Model file for the job. Use its own axes, mm. Coordinates: 2 decimals unless noted, no trailing zeros. Order: outer loops, then holes, each group sorted by start corner. A loop starts at its lowest first (then second) coordinate and runs counter-clockwise, first axis right, second up. Notation, with made-up numbers: M -10.75,-9.5 L 0.25,-9.5 A36 cw 0.25,28.5 Z; hole C -16,46.25 d2. An arc over 180 degrees is marked long. Return JSON: item names as keys, results as strings.
```python
from build123d import *

# Parameters (mm, degrees)
ESBO_O1_W                                            = 18
ESBO_O1_H                                            = 400
RESSALTO_EXTRUS_O1_DEPTH                             = 3.5
FURO_DE_DI_METRO_2_0_2_1_D                           = 2
FURO_DE_DI_METRO_6_0_6_1_D                           = 6
REBAIXO_PARA_PARAFUSO_DE_M_QUINA_DE_CABE_D           = 3.5
REBAIXO_PARA_PARAFUSO_DE_M_QUINA_DE_CABE_CBORE_D     = 6
REBAIXO_PARA_PARAFUSO_DE_M_QUINA_DE_CABE_CBORE_DEPTH = 3.5
PADR_O_LINEAR1_COUNT                                 = 13
PADR_O_LINEAR1_PITCH                                 = 30
PADR_O_LINEAR2_COUNT                                 = 14
PADR_O_LINEAR2_PITCH                                 = 30
CHANFRO1_SIZE                                        = 0.3


with BuildPart() as part:
    # Esboço1 → Ressalto-extrusão1 (new, symmetric)
    with BuildSketch(Plane.XZ):
        Rectangle(ESBO_O1_W, ESBO_O1_H)
    extrude(amount=RESSALTO_EXTRUS_O1_DEPTH, both=True)

    # Furo de diâmetro Ø2.0 (2)1 (through all)
    with Locations(Plane(origin=(0, 0, -200), x_dir=(-1, 0, 0), z_dir=(0, 0, -1))):
        with Locations((-8.669077014, 4.635653864), (9, 1.2)):
            furo_de_di_metro_2_0_2_1 = Hole(FURO_DE_DI_METRO_2_0_2_1_D / 2)

    # Furo de diâmetro Ø6.0 (6)1 (through all)
    with Locations(Plane(origin=(0, 3.5, 0), x_dir=(1, 0, 0), z_dir=(0, 1, 0))):
        with Locations((0, -175)):
            furo_de_di_metro_6_0_6_1 = Hole(FURO_DE_DI_METRO_6_0_6_1_D / 2)

    # Rebaixo para parafuso de máquina de cabeça sextavada de M31 (through all)
    with Locations(Plane(origin=(0, 3.5, 0), x_dir=(1, 0, 0), z_dir=(0, 1, 0))):
        with Locations((0, -190)):
            rebaixo_para_parafuso_de_m_quina_de_cabe = CounterBoreHole(REBAIXO_PARA_PARAFUSO_DE_M_QUINA_DE_CABE_D / 2, REBAIXO_PARA_PARAFUSO_DE_M_QUINA_DE_CABE_CBORE_D / 2, REBAIXO_PARA_PARAFUSO_DE_M_QUINA_DE_CABE_CBORE_DEPTH)

    # Padrão linear1: Furo de diâmetro Ø6.0 (6)1 ×13
    with Locations(*[(0, 0, -i * PADR_O_LINEAR1_PITCH) for i in range(1, PADR_O_LINEAR1_COUNT)]):
        add(furo_de_di_metro_6_0_6_1, mode=Mode.SUBTRACT)

    # Padrão linear2: Rebaixo para parafuso de máquina de cabeça sextavada de M31 ×14
    with Locations(*[(0, 0, -i * PADR_O_LINEAR2_PITCH) for i in range(1, PADR_O_LINEAR2_COUNT)]):
        add(rebaixo_para_parafuso_de_m_quina_de_cabe, mode=Mode.SUBTRACT)

    # Chanfro1
    chanfro1_edges = [part.edges().sort_by_distance(p)[0] for p in [
        (9, 3.5, 0),
        (-9, 3.5, 0),
        (9, -3.5, 0),
        (-9, -3.5, 0),
    ]]
    chamfer(chanfro1_edges, length=CHANFRO1_SIZE)

    # Mirror1: Furo de diâmetro Ø2.0 (2)1 across plane
    add(furo_de_di_metro_2_0_2_1.mirror(Plane(origin=(0, 0, 0), x_dir=(0, 0, 1), z_dir=(1, 0, 0))), mode=Mode.SUBTRACT)


solid = part.part
```
Item 1: Wall check: line 1 (X direction, y = 1, z = -110); line 2 (X direction, y = -0.75, z = 70); line 3 (X direction, y = 1, z = -1). Give the ranges that are in metal, low to high.
Check result:
{"line 1": "x = -8.02 to -3, 3 to 8.02", "line 2": "x = -9 to -1.75, 1.75 to 9", "line 3": "x = -8.02 to 8.02"}
Item 2: Drop flat-ended pins along their axis: pin 1 Ø5 at (x, z) = (0, 145) entering from +Y; pin 2 Ø4.5 at (x, z) = (0, 130) entering from +Y. Give the stop position or say it passes through.
Check result:
{"pin 1": "passes through", "pin 2": "stops at y = 0"}
Item 3: Saw through at A-A (z = -162). Write the cut outline in (x, y).
Check result:
{"outline": "M -9,-3.2 L -8.7,-3.5 L 8.7,-3.5 L 9,-3.2 L 9,0.2 A1 cw 9,2.2 L 9,3.2 L 8.7,3.5 L -8.7,3.5 L -9,3.2 L -9,2.2 A1 cw -9,0.2 Z"}
